```python
from build123d import *

# Parameters (mm, degrees)
EXTRUDE1_DEPTH         = 6.35
M4X0_7_TAPPED_HOLE1_D  = 3.3
F_10_CLEARANCE_HOLE1_D = 5.6134


with BuildPart() as part:
    # Sketch1 → Extrude1 (new, symmetric)
    with BuildSketch(Plane(origin=(0, 0, 0), x_dir=(1, 0, 0), z_dir=(0, 1, 0))):
        Polygon((47.625, 0), (53.848, 0), (53.848, -2.54), (60.325, -2.54), (60.325, -12.7), (41.275, -12.7), (41.275, -38.1), (30.1625, -38.1), (30.1625, -12.7), (11.1125, -12.7), (11.1125, -38.1), (0, -38.1), (0, -2.54), (47.625, -2.54), align=None)
    extrude(amount=EXTRUDE1_DEPTH, both=True)

    # M4x0.7 Tapped Hole1 (through all)
    with Locations(Plane(origin=(41.275, 0, 0), x_dir=(0, 0, -1), z_dir=(1, 0, 0))):
        with Locations((-31.75, 0)):
            Hole(M4X0_7_TAPPED_HOLE1_D / 2)

    # #10 Clearance Hole1 (through all)
    with Locations(Plane(origin=(0, 0, 0), x_dir=(-1, 0, 0), z_dir=(0, 0, -1))):
        with Locations((-50.7365, 0)):
            Hole(F_10_CLEARANCE_HOLE1_D / 2)


solid = part.part
```
Geometry check sheet. Reference: the model listing, model coordinates, mm. A direction names the side the tool comes from. Round coordinates to 2 decimals unless told otherwise and drop trailing zeros. Write item = value, one per line. Start each with the question number.
1. Depth check by flat-ended pin: pin 1 (4 mm diameter, centred on y = -2, z = 20.5, fed in from -X); pin 2 (6.5 mm diameter, centred on x = 13.5, y = 2, fed in from -Z); pin 3 (2 mm diameter, centred on y = -2, z = 1, fed in from +X); pin 4 (6.5 mm diameter, centred on x = 16, y = 2.5, fed in from +Z). Enter the tip coordinate at first touch or a pass-through.
2. Thickness scan on line 1 (Y direction, x = 7.5, z = 31.75); line 2 (X direction, y = -2, z = 26) (1 decimal); line 3 (Z direction, x = 22.5, y = 3.75). Record the ranges inside material, lowest first.
3. Section check B-B on z = 31.75. Give the number of separate pieces and of enclosed holes in the cut face, then the cut area to 3 significant figures.
4. Mould release check, pull along Z, two halves, no side actions. Record for faces 4 (the face through (47.625, 0, 1)), 5 (the face through (36, 0, 38.1)), 6 (the face through (35.64, 0.07, 30.1)): released by +Z, released by -Z, zero draft, split by the parting line, or undercut.
5. Set-up check for faces 1 (the face through (53.848, 0, 1)), 2 (the face through (23, 0, 2.54)), 3 (the face through (41.275, 0, 25)): record each of +Z, -Z, +X, -X, +Y, -Y from which the full face is reachable in a straight line by a thin tool's end or side.
Working result:
q1.pin_1 = 0
q1.pin_2 = 2.54
q1.pin_3 = 53.85
q1.pin_4 = 12.7
q2.line_1 = -6.35 to -1.65, 1.65 to 6.35
q2.line_2 = 0 to 11.1, 30.2 to 41.3
q2.line_3 = 2.54 to 12.7
q3.separate_pieces = 4
q3.enclosed_holes = 0
q3.area = 209 mm^2
q4.face_4 = zero draft
q4.face_5 = released by +Z
q4.face_6 = undercut
q5.face_1 = -Z, +X, +Y, -Y
q5.face_2 = -Z, -X, +Y, -Y
q5.face_3 = +Z, +X, +Y, -Y
